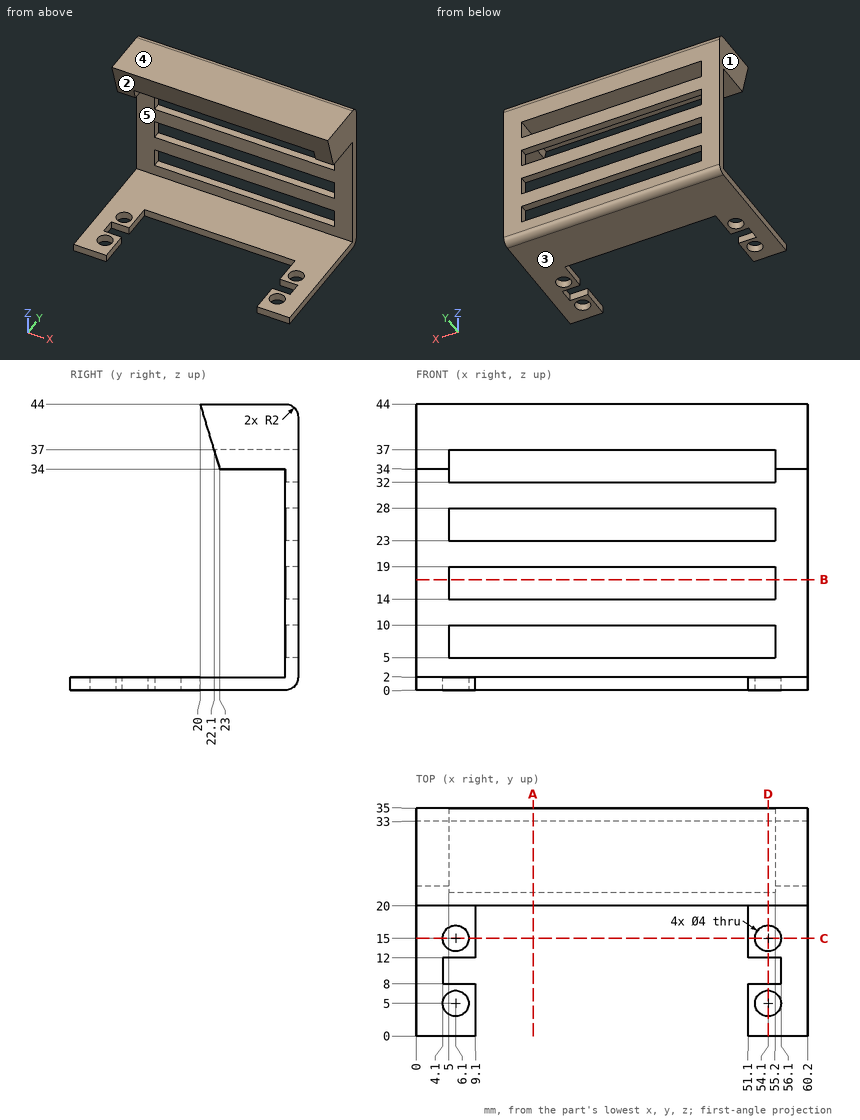
Answer from the drawing. Dimensions are ordinates in mm from the lowest x, y and z of the part. A direction names the side the tool comes from. Give positions to 0.01 mm unless a question says otherwise; leave off trailing zeros. Loops run counter-clockwise (first coordinate to the right, second up) from the corner with the lowest first, then second, coordinate; pieces in that order, holes last. Notation, with made-up numbers: (37.5, 23.5) -> (91.5, 23.5) arc R12 ccw to (91.5, 29.5) -> close; hole circle Ø6 at (15, 55). An arc over 180 degrees is marked (long way). Answer as CSV lines item,"result".
Item 1: Find section C-C on y = 15. Give the vertices of the cut face in (x, z).
Returned:
outline,"(0, 0) -> (4.1, 0) -> (4.1, 2) -> (0, 2) -> close; (8.1, 0) -> (9.1, 0) -> (9.1, 2) -> (8.1, 2) -> close; (51.1, 0) -> (52.1, 0) -> (52.1, 2) -> (51.1, 2) -> close; (56.1, 0) -> (60.2, 0) -> (60.2, 2) -> (56.1, 2) -> close"
Item 2: For the marked faces 1 and 2, determine the directions among +Z, -Z, +X, -X, +Y, -Y from which every point of the face is accessible in a straight line to the end or side of a thin tool.
Returned:
face 1,"+Z, -Z, -X, +Y, -Y"
face 2,"+X, -X, -Y"
Item 3: Each of these flat-tipped pins is pushed along its axis until it touches: pin 1 (5.5 mm diameter, centred on x = 1.5, y = 29, fed in from -Z); pin 2 (0.6 mm diameter, centred on x = 35, y = 34, fed in from -Z); pin 3 (2 mm diameter, centred on x = 25, y = 34.5, fed in from +Z); pin 4 (1 mm diameter, centred on x = 5.5, z = 1, fed in from +Y). Where does it stop, or does it pass through?
Returned:
pin 1,"stops at z = 0"
pin 2,"stops at z = 0.13"
pin 3,"stops at z = 43.94"
pin 4,"stops at y = 34.94"
Item 4: Find section A-A on x = 18. Give the vertices of the cut face in (y, z), plus the area to 3 significant figures.
Returned:
outline,"(20, 0) -> (33, 0) arc R2 ccw to (35, 2) -> (35, 5) -> (33, 5) -> (33, 2) -> (20, 2) -> close; (20, 44) -> (22.1, 37) -> (35, 37) -> (35, 42) arc R2 ccw to (33, 44) -> close; (33, 10) -> (35, 10) -> (35, 14) -> (33, 14) -> close; (33, 19) -> (35, 19) -> (35, 23) -> (33, 23) -> close; (33, 28) -> (35, 28) -> (35, 32) -> (33, 32) -> close"
area,"156 mm²"
Item 5: Find section D-D on x = 54.1. State how many separate pieces and enclosed holes the cut face has, plus the area to 3 significant figures.
Returned:
separate pieces,"8"
enclosed holes,"0"
area,"172 mm²"
Item 6: Consider line 1 (Z direction, x = 40, y = 28); line 2 (Y direction, x = 32.5, z = 21); line 3 (Z direction, x = 7.5, y = 33.5). Determine where each line is inside the solid, lowest interval first. Write a range as [from, to].
Returned:
line 1,"z = [0, 2], [37, 44]"
line 2,"y = [33, 35]"
line 3,"z = [0.06, 5], [10, 14], [19, 23], [28, 32], [37, 43.94]"
Item 7: Find section B-B on z = 17. Give the vertices of the cut face in (x, y).
Returned:
outline,"(0, 33) -> (5, 33) -> (5, 35) -> (0, 35) -> close; (55.2, 33) -> (60.2, 33) -> (60.2, 35) -> (55.2, 35) -> close"
Item 8: Determine the mould class of the marked faces 3, 4 and 5 for opening direction Z: +Z half, -Z half, draft (parallel to the pull), parting line (faces both ways), or undercut.
Returned:
face 3,"-Z half"
face 4,"+Z half"
face 5,"undercut"
